Answer from the drawing. Dimensions are ordinates in mm from the lowest x, y and z of the part. A direction names the side the tool comes from. Give positions to 0.01 mm unless a question says otherwise; leave off trailing zeros. Loops run counter-clockwise (first coordinate to the right, second up) from the corner with the lowest first, then second, coordinate; pieces in that order, holes last. Notation, with made-up numbers: (24, 30.25) -> (39, 30.25) arc R18 cw to (39, 55.25) -> close; hole circle Ø7 at (-17.75, 14.25). An arc over 180 degrees is marked (long way). Return JSON: item names as keys, results as strings. Group by question number.
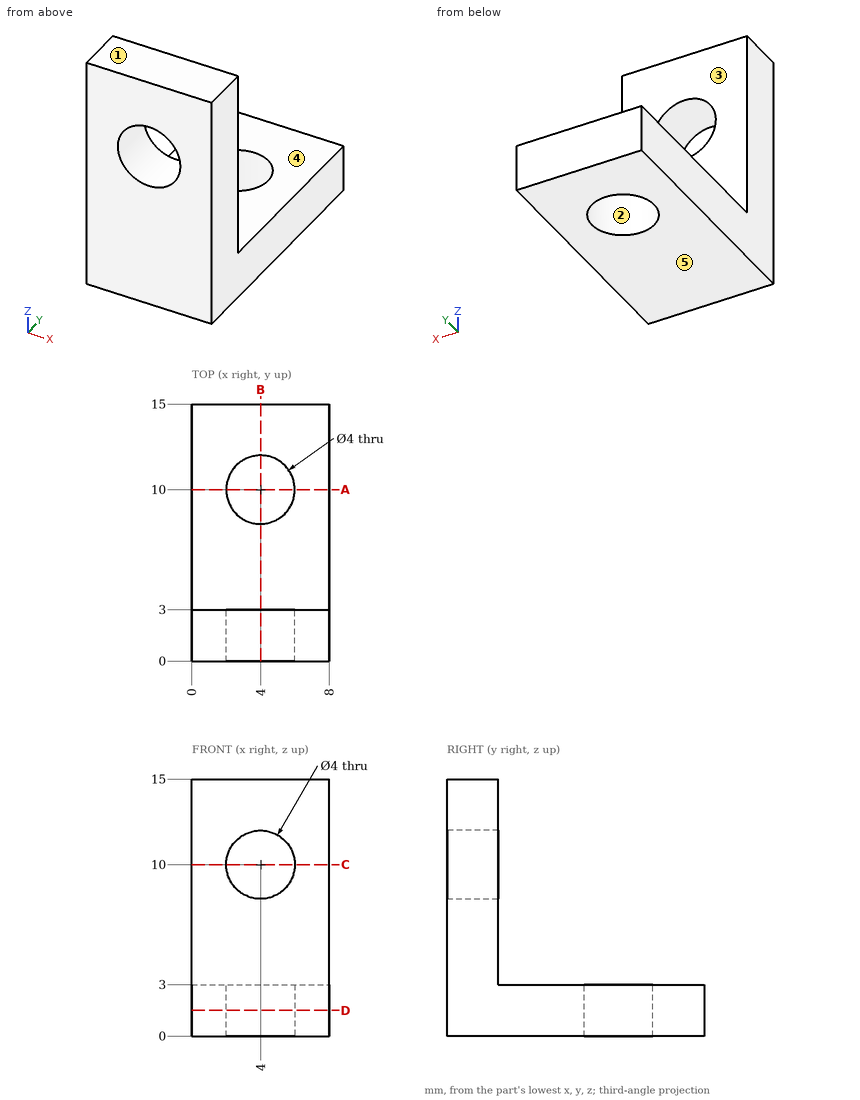
1. Section D-D on z = 1.5 is taken. Determine the outline of the cut face in (x, y).
2. Determine the mould class of the marked faces 1, 2 and 3 for opening direction Y: pulls with the +Y half, pulls with the -Y half, needs draft (parallel to the pull), parting line crosses it, or undercut.
3. Section A-A on y = 10 is taken. Determine the outline of the cut face in (x, z), then the cut area to 3 significant figures.
4. Straight lines are drawn through the part: line 1 (Y direction, x = 4, z = 2.4); line 2 (X direction, y = 1.3, z = 10); line 3 (Z direction, x = 2.25, y = 7.25). For each, find the intervals that lie inside material, in ascending order. Write a range as from..to.
5. Section B-B on x = 4 is taken. Determine the outline of the cut face in (y, z).
6. Which of the six approach directions +Z, -Z, +X, -X, +Y, -Y give full straight-line access (tool end or side, diameter ignored) to the marked faces 4 and 5?
Completed:
{
 "1": {"outline": "(0, 0) -> (8, 0) -> (8, 15) -> (0, 15) -> close; hole circle Ø4 at (4, 10)"},
 "2": {"face 1": "needs draft", "face 2": "undercut", "face 3": "pulls with the +Y half"},
 "3": {"outline": "(0, 0) -> (2, 0) -> (2, 3) -> (0, 3) -> close; (6, 0) -> (8, 0) -> (8, 3) -> (6, 3) -> close", "area": "12.0 mm²"},
 "4": {"line 1": "y = 0..8, 12..15", "line 2": "x = 0..2, 6..8", "line 3": "z = 0..3"},
 "5": {"outline": "(0, 0) -> (8, 0) -> (8, 3) -> (3, 3) -> (3, 8) -> (0, 8) -> close; (0, 12) -> (3, 12) -> (3, 15) -> (0, 15) -> close; (12, 0) -> (15, 0) -> (15, 3) -> (12, 3) -> close"},
 "6": {"face 4": "+Z, +X, -X, +Y", "face 5": "-Z, +X, -X, +Y, -Y"}
}
